Design review of the part built by this model. Coordinates are the model's own, in mm. A direction names the side the tool comes from. Round coordinates to 2 decimals unless told otherwise and drop trailing zeros. Write each loop counter-clockwise with the first axis right and the second up, starting at its lowest first coordinate (ties: lowest second). Pieces come first, ordered by that corner, then holes. Notation, with made-up numbers: (85, 59) -> (105, 59) arc R33 cw to (105, 91) -> close; hole circle Ø9 at (39.25, 5). An arc over 180 degrees is marked (long way). One line per question, with ' | ' between items. Start each with the question number.
1) Insertion check: pin 1 Ø7.5 at (x, y) = (-4, 6) entering from +Z; pin 2 Ø1 at (x, y) = (0, -10) entering from +Z. Each pin has a flat end and moves straight along its axis. Give the tip position at first contact, or say it passes through.
2) Consider section B-B (z = 17.75). Give the boundary of the cut face in (x, y).
3) For probe 1 along X at (y, z) = (2, 17.5); probe 2 along X at (y, z) = (-8, 9.25), list the stretches that pass through material, from the lowest coordinate up.
4) Mouldability with a two-part tool opening along Y and no side actions: class faces 3 (the flat face through (13.18, 16.19, 16.97)), 4 (the flat face through (18, 0, 9)) as +Y half, -Y half, draft (parallel to the pull), parting line (faces both ways), or undercut.
5) Consider section A-A (x = -8). Give the boundary of the cut face in (y, z), then the cut area to 3 significant figures.
6) Consider section D-D (z = 5.25). Count the separate pieces of the cut face and the enclosed holes in it, then the cut area to 3 significant figures.
7) Consider section C-C (y = -6). Give the boundary of the cut face in (x, z).
8) For faces 1 (the flat face through (0, 0, -0.2)), 2 (the flat face through (-5.34, -14.33, 7.4)), list the 3-axis set-ups (+Z, -Z, +X, -X, +Y, -Y) from which the entire face can be reached by the end or side of a thin tool; tool diameter is ignored.
Autodesk Fusion 360 part; units mm, degrees
sketch "8x8_led_matrix_display" plane through (0, 0, 0) normal (0, 0, 1) x (1, 0, 0)
  circle A0 centre (-14, 14) radius 1.5
  circle A1 centre (-10, 14) radius 1.5
  circle A2 centre (-6, 14) radius 1.5
  circle A3 centre (-2, 14) radius 1.5
  circle A4 centre (2, 14) radius 1.5
  circle A5 centre (6, 14) radius 1.5
  circle A6 centre (10, 14) radius 1.5
  circle A7 centre (14, 14) radius 1.5
  circle A8 centre (-14, 10) radius 1.5
  circle A9 centre (-10, 10) radius 1.5
  circle A10 centre (-6, 10) radius 1.5
  circle A11 centre (-2, 10) radius 1.5
  circle A12 centre (2, 10) radius 1.5
  circle A13 centre (6, 10) radius 1.5
  circle A14 centre (10, 10) radius 1.5
  circle A15 centre (14, 10) radius 1.5
  circle A16 centre (-14, 6) radius 1.5
  circle A17 centre (-10, 6) radius 1.5
  circle A18 centre (-6, 6) radius 1.5
  circle A19 centre (-2, 6) radius 1.5
  circle A20 centre (2, 6) radius 1.5
  circle A21 centre (6, 6) radius 1.5
  circle A22 centre (10, 6) radius 1.5
  circle A23 centre (14, 6) radius 1.5
  circle A24 centre (-14, 2) radius 1.5
  circle A25 centre (-10, 2) radius 1.5
  circle A26 centre (-6, 2) radius 1.5
  circle A27 centre (-2, 2) radius 1.5
  circle A28 centre (2, 2) radius 1.5
  circle A29 centre (6, 2) radius 1.5
  circle A30 centre (10, 2) radius 1.5
  circle A31 centre (14, 2) radius 1.5
  circle A32 centre (-14, -2) radius 1.5
  circle A33 centre (-10, -2) radius 1.5
  circle A34 centre (-6, -2) radius 1.5
  circle A35 centre (-2, -2) radius 1.5
  circle A36 centre (2, -2) radius 1.5
  circle A37 centre (6, -2) radius 1.5
  circle A38 centre (10, -2) radius 1.5
  circle A39 centre (14, -2) radius 1.5
  circle A40 centre (-14, -6) radius 1.5
  circle A41 centre (-10, -6) radius 1.5
  circle A42 centre (-6, -6) radius 1.5
  circle A43 centre (-2, -6) radius 1.5
  circle A44 centre (2, -6) radius 1.5
  circle A45 centre (6, -6) radius 1.5
  circle A46 centre (10, -6) radius 1.5
  circle A47 centre (14, -6) radius 1.5
  circle A48 centre (-14, -10) radius 1.5
  circle A49 centre (-10, -10) radius 1.5
  circle A50 centre (-6, -10) radius 1.5
  circle A51 centre (-2, -10) radius 1.5
  circle A52 centre (2, -10) radius 1.5
  circle A53 centre (6, -10) radius 1.5
  circle A54 centre (10, -10) radius 1.5
  circle A55 centre (14, -10) radius 1.5
  circle A56 centre (-14, -14) radius 1.5
  circle A57 centre (-10, -14) radius 1.5
  circle A58 centre (-6, -14) radius 1.5
  circle A59 centre (-2, -14) radius 1.5
  circle A60 centre (2, -14) radius 1.5
  circle A61 centre (6, -14) radius 1.5
  circle A62 centre (10, -14) radius 1.5
  circle A63 centre (14, -14) radius 1.5
  line L0 (16, -16) -> (-16, -16)
  line L1 (-16, -16) -> (-16, 16)
  line L2 (-16, 16) -> (16, 16)
  line L3 (16, 16) -> (16, -16)
  line L4 (16, -16) -> (-16, 16) construction
  line L5 (-16, -16) -> (16, 16) construction
  line L6 (18, -18) -> (-18, -18)
  line L7 (-18, -18) -> (-18, 18)
  line L8 (-18, 18) -> (18, 18)
  line L9 (18, 18) -> (18, -18)
  dimension "d1" = 3
  dimension "d2" = 14
  dimension "d3" = 14
  dimension "d6" = 28
  dimension "d7" = -28
  dimension "d8" = 32
  dimension "d9" = 32
  dimension "d33" = -2
sketch "segments" plane through (0, 0, 0) normal (0, 0, 1) x (1, 0, 0)
  line L0 (0, 0) -> (-16, 0)
  line L1 (-16, 0) -> (-16, 16)
  line L2 (-16, 16) -> (0, 16)
  line L3 (0, 16) -> (0, 0)
  line L4 (-11.5, 0) -> (-11.5, 8.1712)
  line L5 (-11.5, 8.1712) -> (-8.5, 11.1712)
  line L6 (-8.5, 11.1712) -> (-8.5, 0)
  line L7 (-7.5, 12.1712) -> (-7.5, 3.961)
  line L8 (-7.5, 3.961) -> (-2.5572, 0.5)
  line L9 (-2.5572, 0.5) -> (-0.5, 0.5)
  line L10 (-0.5, 0.5) -> (-0.5, 2.7218)
  line L11 (-0.5, 2.7218) -> (-4.5, 5.5227)
  line L12 (-4.5, 5.5227) -> (-4.5, 10.5993)
  line L13 (-4.5, 10.5993) -> (-7.189, 12.4822)
  line L14 (-7.189, 12.4822) -> (-7.5, 12.1712)
  line L15 (0, 11.5) -> (-1.5, 11.5)
  line L16 (-1.5, 11.5) -> (-1.5, 4.6428)
  line L17 (-1.5, 4.6428) -> (0, 3.5925)
  line L18 (0, 15.5) -> (-4.1712, 15.5)
  line L19 (-4.1712, 15.5) -> (-6.471, 13.2002)
  line L20 (-6.471, 13.2002) -> (-5.471, 12.5)
  line L21 (-5.471, 12.5) -> (0, 12.5)
  dimension "d10" = 16
  dimension "d11" = 16
  dimension "d12" = 3
  dimension "d13" = 8.5
  dimension "d14" = 3
  dimension "d15" = 3
  dimension "d16" = 0.5
  dimension "d17" = 0.5
  dimension "d18" = 1
  dimension "d19" = 1.5
  dimension "d20" = 11.5
  dimension "d21" = 1
  dimension "d22" = 3
  dimension "d23" = 15.5
  dimension "d24" = 1
  dimension "d25" = 45
  dimension "d26" = 125
extrude "Extrude1" add sketch "segments" along normal blind 15 contours L0 L1 L2 L3 L4 L5 L6 L15 L16 L17 L18 L19 L20 L21
mirror "Mirror1" about plane through (0, 0, 0) normal (1, 0, 0) of bodies 1 merged
mirror "Mirror2" about plane through (0, 0, 0) normal (0, 1, 0) of bodies 1 merged
extrude "Extrude2" add sketch "8x8_led_matrix_display" along normal blind 15 contours L6 L7 L8 L9
fillet "Fillet1" radius 2 4 edges at (-18, -18, 7.5) (18, -18, 7.5) (18, 18, 7.5) (-18, 18, 7.5)
sketch "projected_for_diffuser" plane through (0, 0, 0) normal (0, 0, -1) x (1, 0, 0)
  arc A0 (-18, -16) -> (-16, -18) centre (-16, -16) ccw
  line L0 (-16, -18) -> (16, -18)
  arc A1 (16, -18) -> (18, -16) centre (16, -16) ccw
  line L1 (18, -16) -> (18, 16)
  arc A2 (18, 16) -> (16, 18) centre (16, 16) ccw
  line L2 (16, 18) -> (-16, 18)
  arc A3 (-16, 18) -> (-18, 16) centre (-16, 16) ccw
  line L3 (-18, 16) -> (-18, -16)
  line L4 (11.5, 8.1712) -> (11.5, -8.1712)
  line L5 (11.5, -8.1712) -> (8.5, -11.1712)
  line L6 (8.5, -11.1712) -> (8.5, 11.1712)
  line L7 (8.5, 11.1712) -> (11.5, 8.1712)
  line L8 (-7.5, 12.1712) -> (-7.189, 12.4822)
  line L9 (-7.189, 12.4822) -> (-4.5, 10.5993)
  line L10 (-4.5, 10.5993) -> (-4.5, 5.5227)
  line L11 (-4.5, 5.5227) -> (-0.5, 2.7218)
  line L12 (-0.5, 2.7218) -> (-0.5, 0.5)
  line L13 (-0.5, 0.5) -> (-2.5572, 0.5)
  line L14 (-2.5572, 0.5) -> (-7.5, 3.961)
  line L15 (-7.5, 3.961) -> (-7.5, 12.1712)
  line L16 (7.189, 12.4822) -> (7.5, 12.1712)
  line L17 (7.5, 12.1712) -> (7.5, 3.961)
  line L18 (7.5, 3.961) -> (2.5572, 0.5)
  line L19 (2.5572, 0.5) -> (0.5, 0.5)
  line L20 (0.5, 0.5) -> (0.5, 2.7218)
  line L21 (0.5, 2.7218) -> (4.5, 5.5227)
  line L22 (4.5, 5.5227) -> (4.5, 10.5993)
  line L23 (4.5, 10.5993) -> (7.189, 12.4822)
  line L24 (-1.5, 11.5) -> (1.5, 11.5)
  line L25 (1.5, 11.5) -> (1.5, 4.6428)
  line L26 (1.5, 4.6428) -> (0, 3.5925)
  line L27 (0, 3.5925) -> (-1.5, 4.6428)
  line L28 (-1.5, 4.6428) -> (-1.5, 11.5)
  line L29 (-4.1712, 15.5) -> (4.1712, 15.5)
  line L30 (4.1712, 15.5) -> (6.471, 13.2002)
  line L31 (6.471, 13.2002) -> (5.471, 12.5)
  line L32 (5.471, 12.5) -> (-5.471, 12.5)
  line L33 (-5.471, 12.5) -> (-6.471, 13.2002)
  line L34 (-6.471, 13.2002) -> (-4.1712, 15.5)
  line L35 (4.1712, -15.5) -> (-4.1712, -15.5)
  line L36 (-4.1712, -15.5) -> (-6.471, -13.2002)
  line L37 (-6.471, -13.2002) -> (-5.471, -12.5)
  line L38 (-5.471, -12.5) -> (5.471, -12.5)
  line L39 (5.471, -12.5) -> (6.471, -13.2002)
  line L40 (6.471, -13.2002) -> (4.1712, -15.5)
  line L41 (1.5, -11.5) -> (-1.5, -11.5)
  line L42 (-1.5, -11.5) -> (-1.5, -4.6428)
  line L43 (-1.5, -4.6428) -> (0, -3.5925)
  line L44 (0, -3.5925) -> (1.5, -4.6428)
  line L45 (1.5, -4.6428) -> (1.5, -11.5)
  line L46 (7.5, -12.1712) -> (7.189, -12.4822)
  line L47 (7.189, -12.4822) -> (4.5, -10.5993)
  line L48 (4.5, -10.5993) -> (4.5, -5.5227)
  line L49 (4.5, -5.5227) -> (0.5, -2.7218)
  line L50 (0.5, -2.7218) -> (0.5, -0.5)
  line L51 (0.5, -0.5) -> (2.5572, -0.5)
  line L52 (2.5572, -0.5) -> (7.5, -3.961)
  line L53 (7.5, -3.961) -> (7.5, -12.1712)
  line L54 (-7.189, -12.4822) -> (-7.5, -12.1712)
  line L55 (-7.5, -12.1712) -> (-7.5, -3.961)
  line L56 (-7.5, -3.961) -> (-2.5572, -0.5)
  line L57 (-2.5572, -0.5) -> (-0.5, -0.5)
  line L58 (-0.5, -0.5) -> (-0.5, -2.7218)
  line L59 (-0.5, -2.7218) -> (-4.5, -5.5227)
  line L60 (-4.5, -5.5227) -> (-4.5, -10.5993)
  line L61 (-4.5, -10.5993) -> (-7.189, -12.4822)
  line L62 (-11.5, -8.1712) -> (-11.5, 8.1712)
  line L63 (-11.5, 8.1712) -> (-8.5, 11.1712)
  line L64 (-8.5, 11.1712) -> (-8.5, -11.1712)
  line L65 (-8.5, -11.1712) -> (-11.5, -8.1712)
extrude "Extrude3" add sketch "projected_for_diffuser" along normal blind 0.2 contours A0 L0 A1 L1 A2 L2 A3 L3 | L4 L5 L6 L7 | L8 L9 L10 L11 L12 L13 L14 L15 | L16 L17 L18 L19 L20 L21 L22 L23 | L24 L25 L26 L27 L28 | L29 L30 L31 L32 L33 L34 | L35 L36 L37 L38 L39 L40 | L41 L42 L43 L44 L45 | L46 L47 L48 L49 L50 L51 L52 L53 | L54 L55 L56 L57 L58 L59 L60 L61 | L62 L63 L64 L65
sketch "grip_for_display" plane through (0, 0, 15) normal (0, 0, 1) x (-1, 0, 0)
  line L0 (16, -16) -> (-16, -16)
  line L1 (-16, -16) -> (-16, 16)
  line L2 (-16, 16) -> (16, 16)
  line L3 (16, 16) -> (16, -16)
  line L4 (16, -16) -> (-16, 16) construction
  line L5 (-16, -16) -> (16, 16) construction
  line L6 (16, -11) -> (-16, -11)
  line L7 (-16, -11) -> (-16, 11)
  line L8 (-16, 11) -> (16, 11)
  line L9 (16, 11) -> (16, -11)
  line L10 (16, -11) -> (-16, 11) construction
  line L11 (-16, -11) -> (16, 11) construction
  line L12 (11, -16) -> (-11, -16)
  line L13 (-11, -16) -> (-11, 16)
  line L14 (-11, 16) -> (11, 16)
  line L15 (11, 16) -> (11, -16)
  line L16 (11, -16) -> (-11, 16) construction
  line L17 (-11, -16) -> (11, 16) construction
  line L18 (-16, 11) -> (-16.4794, 16.4794)
  line L19 (-16.4794, 16.4794) -> (-11, 16)
  line L20 (11, 16) -> (16.4794, 16.4794)
  line L21 (16.4794, 16.4794) -> (16, 11)
  line L22 (16, -11) -> (16.4794, -16.4794)
  line L23 (16.4794, -16.4794) -> (11, -16)
  line L24 (-16, -11) -> (-16.4794, -16.4794)
  line L25 (-16.4794, -16.4794) -> (-11, -16)
  line L26 (-16, -18) -> (16, -18)
  arc A0 (-18, -16) -> (-16, -18) centre (-16, -16) ccw
  line L27 (-18, 16) -> (-18, -16)
  arc A1 (-16, 18) -> (-18, 16) centre (-16, 16) ccw
  line L28 (16, 18) -> (-16, 18)
  arc A2 (18, 16) -> (16, 18) centre (16, 16) ccw
  line L29 (18, -16) -> (18, 16)
  arc A3 (16, -18) -> (18, -16) centre (16, -16) ccw
  dimension "d40" = 32
  dimension "d41" = 32
  dimension "d42" = 32
  dimension "d43" = 22
  dimension "d44" = 22
  dimension "d45" = 32
  dimension "d46" = 80
extrude "Extrude4" add sketch "grip_for_display" along normal blind 4
fillet "Fillet2" radius 1 4 edges at (16.4794, -16.4794, 17) (-16.4794, -16.4794, 17) (-16.4794, 16.4794, 17) (16.4794, 16.4794, 17)
fillet "Fillet2" radius 5 8 edges at (16, -11, 17) (11, -16, 17) (-11, -16, 17) (-16, -11, 17) (-16, 11, 17) (-11, 16, 17) (11, 16, 17) (16, 11, 17)
equation "d2 = ( 3.5 * 4 ) * 1 mm"
equation "d3 = ( 3.5 * 4 ) * 1 mm"
equation "d6 = ( 4 * 7 ) * 1 mm"
equation "d7 = ( -4 * 7 ) * 1 mm"
From the geometry:
1) pin 1: stops at z = 15 | pin 2: stops at z = 0
2) outline: (-18, -16) arc R2 ccw to (-16, -18) -> (16, -18) arc R2 ccw to (18, -16) -> (18, 16) arc R2 ccw to (16, 18) -> (-16, 18) arc R2 ccw to (-18, 16) -> close; hole (-16.38, -15.29) arc R1 ccw to (-15.29, -16.38) -> (-11, -16) -> (11, -16) -> (15.29, -16.38) arc R1 ccw to (16.38, -15.29) -> (16, -11) -> (16, 11) -> (16.38, 15.29) arc R1 ccw to (15.29, 16.38) -> (11, 16) -> (-11, 16) -> (-15.29, 16.38) arc R1 ccw to (-16.38, 15.29) -> (-16, 11) -> (-16, -11) -> close
3) probe 1: x = -18 to -16, 16 to 18 | probe 2: x = -18 to -11.5, -8.5 to -7.5, -4.5 to -1.5, 1.5 to 4.5, 7.5 to 8.5, 11.5 to 18
4) face 3: undercut | face 4: draft
5) outline: (-18, -0.2) -> (18, -0.2) -> (18, 19) -> (16, 19) -> (16, 15) -> (-16, 15) -> (-16, 19) -> (-18, 19) -> close | area: 563 mm2
6) separate pieces: 1 | enclosed holes: 10 | area: 909 mm2
7) outline: (-18, -0.2) -> (18, -0.2) -> (18, 19) -> (16, 19) -> (16, 15) -> (11.5, 15) -> (11.5, 0) -> (8.5, 0) -> (8.5, 15) -> (7.5, 15) -> (7.5, 0) -> (4.5, 0) -> (4.5, 15) -> (1.5, 15) -> (1.5, 0) -> (-1.5, 0) -> (-1.5, 15) -> (-4.5, 15) -> (-4.5, 0) -> (-7.5, 0) -> (-7.5, 15) -> (-8.5, 15) -> (-8.5, 0) -> (-11.5, 0) -> (-11.5, 15) -> (-16, 15) -> (-16, 19) -> (-18, 19) -> close
8) face 1: -Z, +X, -X, +Y, -Y | face 2: +Z
